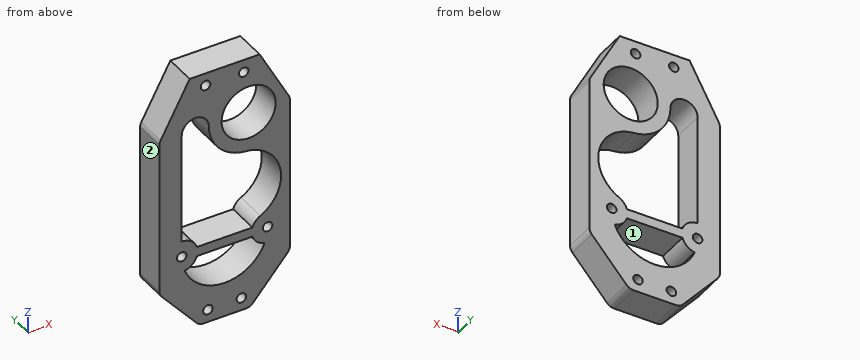
from build123d import *

# Parameters (mm, degrees)
SKETCH1_R           = 1.5
SKETCH1_R_2         = 8.5
BOSS_EXTRUDE1_DEPTH = 5
FILLET1_R           = 3


with BuildPart() as part:
    # Sketch1 → Boss-Extrude1 (new, symmetric)
    with BuildSketch(Plane(origin=(0, 0, 0), x_dir=(1, 0, 0), z_dir=(0, 1, 0))):
        Polygon((8, 24.400284093), (-8, 24.400284093), (-20.5, 10), (-20.5, -40), (-11, -57.599715907), (11, -57.599715907), (20.5, -40), (20.5, 10), align=None)
        with Locations(Location((-5.25, 20.39454584, 0), (0, 0, 270))):
            Circle(SKETCH1_R, mode=Mode.SUBTRACT)
        with Locations(Location((-6, -53.599715907, 0), (0, 0, 270))):
            Circle(SKETCH1_R, mode=Mode.SUBTRACT)
        with Locations(Location((6, -53.599715907, 0), (0, 0, 90))):
            Circle(SKETCH1_R, mode=Mode.SUBTRACT)
        with Locations(Location((5.25, 20.39454584, 0), (0, 0, 90))):
            Circle(SKETCH1_R, mode=Mode.SUBTRACT)
        with Locations(Location((-13.5, 0, 0), (0, 0, 270))):
            Circle(SKETCH1_R, mode=Mode.SUBTRACT)
        with Locations(Location((13.5, 0, 0), (0, 0, 270))):
            Circle(SKETCH1_R, mode=Mode.SUBTRACT)
        with Locations(Location((7.530163354, -39.817414772, 0), (0, 0, 270))):
            Circle(SKETCH1_R_2, mode=Mode.SUBTRACT)
        with BuildLine():
            Line((-13.5, -5), (-13.5, -39.817414772))
            ThreePointArc((-13.5, -39.817414772), (-9.234918323, -44.082496449), (-4.969836646, -39.817414772))
            ThreePointArc((-4.969836646, -39.817414772), (-1.654816501, -31.338845018), (6.531946565, -27.35733599))
            ThreePointArc((6.531946565, -27.35733599), (17.487572325, -17.647670786), (11.187975781, -4.433344563))
            ThreePointArc((11.187975781, -4.433344563), (9.667400631, -3.211102938), (8.730303993, -1.5))
            Line((8.730303993, -1.5), (-8.730303993, -1.5))
            ThreePointArc((-8.730303993, -1.5), (-10.541960108, -4.031128874), (-13.5, -5))
        make_face(mode=Mode.SUBTRACT)
        with BuildLine():
            Line((8.730303993, 1.5), (-8.730303993, 1.5))
            ThreePointArc((-8.730303993, 1.5), (-10.179901517, 3.738575405), (-12.574074074, 4.913518208))
            ThreePointArc((-12.574074074, 4.913518208), (0, 13.5), (12.574074074, 4.913518208))
            ThreePointArc((12.574074074, 4.913518208), (10.179901517, 3.738575405), (8.730303993, 1.5))
        make_face(mode=Mode.SUBTRACT)
    extrude(amount=BOSS_EXTRUDE1_DEPTH, both=True)

    # Fillet1
    fillet1_edges = [part.edges().sort_by_distance(p)[0] for p in [
        (-20.5, 0, 40),
        (-20.5, 0, -10),
        (-8, 0, -24.400284093),
        (8, 0, -24.400284093),
        (20.5, 0, -10),
        (20.5, 0, 40),
    ]]
    fillet(fillet1_edges, radius=FILLET1_R)


solid = part.part
Verification items for the finished model (mm, model axes). Face numbers are marked on the shaded views. A direction names the side the tool comes from. Coordinates: 2 decimals unless noted, no trailing zeros. Loops run counter-clockwise (first coordinate to the right, second up) from the corner with the lowest first, then second, coordinate; pieces in that order, holes last. Notation, with made-up numbers: (55, -4) -> (81, -4) arc R27 ccw to (81, 17) -> close; hole circle Ø1 at (-0.5, -31). An arc over 180 degrees is marked (long way). Answer as a JSON object with one key per item and string values. Group by question number.
Item 1: Sectioned sample at D-D on x = 5.25. Record the boundary of the cut face in (y, z), plus the area to 3 significant figures.
Item 2: Sectioned sample at C-C on y = 3. State how many separate pieces and enclosed holes the cut face has, plus the area to 3 significant figures.
Item 3: Depth check by flat-ended pin: pin 1 (2.5 mm diameter, centred on x = 6, z = 53.6, fed in from +Y); pin 2 (2 mm diameter, centred on x = -13.5, y = 1, fed in from -Z). Enter the tip coordinate at first touch or a pass-through.
Item 4: Scan lines: probe 1 along X at (y, z) = (-4, 15.5); probe 2 along Z at (x, y) = (6, 2.5); probe 3 along Z at (x, y) = (4, 3.5). Record each from-to range of solid material in increasing order.
Item 5: Sectioned sample at A-A on z = 0. Record the boundary of the cut face in (x, y), plus the area to 3 significant figures.
Item 6: Tool access check on the marked faces 1 and 2. Record the directions out of +Z, -Z, +X, -X, +Y, -Y that give a thin tool (end or side, any length) a straight path to the whole face; none if there is none.
Item 7: Sectioned sample at B-B on x = 0.5. Record the boundary of the cut face in (y, z), plus the area to 3 significant figures.
Evaluation:
{
 "1": {"outline": "(-5, -24.4) -> (5, -24.4) -> (5, -21.89) -> (-5, -21.89) -> close; (-5, -18.89) -> (5, -18.89) -> (5, -12.44) -> (-5, -12.44) -> close; (-5, -1.5) -> (5, -1.5) -> (5, 1.5) -> (-5, 1.5) -> close; (-5, 27.53) -> (5, 27.53) -> (5, 31.63) -> (-5, 31.63) -> close; (-5, 48.01) -> (5, 48.01) -> (5, 52.3) -> (-5, 52.3) -> close; (-5, 54.9) -> (5, 54.9) -> (5, 57.6) -> (-5, 57.6) -> close", "area": "231 mm²"},
 "2": {"separate pieces": "1", "enclosed holes": "9", "area": "1,630 mm²"},
 "3": {"pin 1": "passes through", "pin 2": "stops at z = -19.22"},
 "4": {"probe 1": "x = -20.5 to -13.5, 17.73 to 20.5", "probe 2": "z = -24.4 to -21.69, -19.1 to -12.09, -1.5 to 1.5, 27.41 to 31.46, 48.18 to 52.1, 55.1 to 57.6", "probe 3": "z = -24.4 to -21.22, -19.57 to -12.89, -1.5 to 1.5, 27.83 to 32.09, 47.55 to 57.6"},
 "5": {"outline": "(-20.5, -5) -> (-15, -5) -> (-15, 5) -> (-20.5, 5) -> close; (-12, -5) -> (12, -5) -> (12, 5) -> (-12, 5) -> close; (15, -5) -> (20.5, -5) -> (20.5, 5) -> (15, 5) -> close", "area": "350 mm²"},
 "6": {"face 1": "+Y, -Y", "face 2": "+Z, -Z, -X, +Y, -Y"},
 "7": {"outline": "(-5, -24.4) -> (5, -24.4) -> (5, -13.49) -> (-5, -13.49) -> close; (-5, -1.5) -> (5, -1.5) -> (5, 1.5) -> (-5, 1.5) -> close; (-5, 29.48) -> (5, 29.48) -> (5, 35.04) -> (-5, 35.04) -> close; (-5, 44.6) -> (5, 44.6) -> (5, 57.6) -> (-5, 57.6) -> close", "area": "325 mm²"}
}
